Can you work these out from the model? Positions are in its coordinate system, mm. Coordinates: 2 decimals unless noted, no trailing zeros. Loops run counter-clockwise (first coordinate to the right, second up) from the corner with the lowest first, then second, coordinate; pieces in that order, holes last. Notation, with made-up numbers: M 71.25,-14 L 129.25,-14 A27 cw 129.25,2 Z; hole C 59.5,71.25 d3. An arc over 180 degrees is marked long. Answer as a JSON object with one key per item and string values. Group by question number.
Item 1: If I drill on line 1 (Z direction, x = 346.5, y = 205.25); line 2 (Y direction, x = 369, z = 6.75), over which ranges is the centre line in solid material (lowest first)?
Item 2: Suppose I cut it at A-A (y = 194.5). Write out the boundary of the cut face in (x, z).
Item 3: Suppose I cut it at C-C (x = 193). Write out the boundary of the cut face in (y, z), then the cut area to 3 significant figures.
Item 4: Suppose I cut it at B-B (z = 13.75). Write out the boundary of the cut face in (x, y).
```python
from build123d import *

# Parameters (mm, degrees)
SKETCH1_W          = 290
SKETCH1_H          = 20
EXTRUDE1_DEPTH     = 20
SKETCH2_W          = 16
SKETCH2_H          = 16
CUT_EXTRUDE1_DEPTH = 300
SKETCH4_R          = 1.6
CUT_EXTRUDE2_DEPTH = 20


with BuildPart() as part:
    # Sketch1 → Extrude1 (new body)
    with BuildSketch(Plane.XY):
        with Locations((292.497048214, 200.002006631)):
            Rectangle(SKETCH1_W, SKETCH1_H)
    extrude(amount=EXTRUDE1_DEPTH)

    # Sketch2 → Cut-Extrude1 (cut)
    with BuildSketch(Plane.ZY.offset(-147.497048214)):
        with Locations((10, 200.002006631)):
            Rectangle(SKETCH2_W, SKETCH2_H)
    extrude(amount=-CUT_EXTRUDE1_DEPTH, mode=Mode.SUBTRACT)

    # Sketch4 → Cut-Extrude2 (cut)
    with BuildSketch(Plane.XY.offset(20)):
        with Locations((427.497048214, 200.002006631)):
            Circle(SKETCH4_R)
        with Locations((407.497048214, 199.95245399)):
            Circle(SKETCH4_R)
        with Locations((387.497048214, 199.90290135)):
            Circle(SKETCH4_R)
        with Locations((197.497048214, 199.90290135)):
            Circle(SKETCH4_R)
        with Locations((177.497048214, 199.95245399)):
            Circle(SKETCH4_R)
        with Locations((157.497048214, 200.002006631)):
            Circle(SKETCH4_R)
    extrude(amount=-CUT_EXTRUDE2_DEPTH, mode=Mode.SUBTRACT)


solid = part.part
```
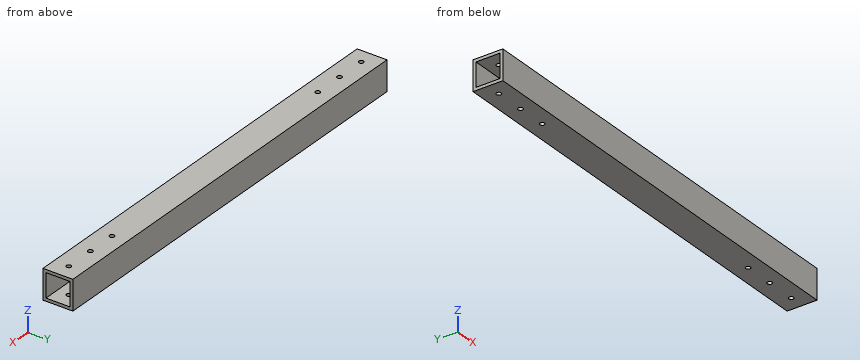
From the geometry:
{
 "1": {"line 1": "0 to 2, 18 to 20", "line 2": "190 to 192, 208 to 210"},
 "2": {"outline": "M 147.5,0 L 437.5,0 L 437.5,2 L 147.5,2 Z; M 147.5,18 L 437.5,18 L 437.5,20 L 147.5,20 Z"},
 "3": {"outline": "M 190,0 L 210,0 L 210,20 L 190,20 Z; hole M 192,2 L 208,2 L 208,18 L 192,18 Z", "area": "144 mm2"},
 "4": {"outline": "M 147.5,190 L 437.5,190 L 437.5,192 L 147.5,192 Z; M 147.5,208 L 437.5,208 L 437.5,210 L 147.5,210 Z"}
}
